Autodesk Inventor part; units mm, degrees
ref_plane "YZ Plane" through (0, 0, 0) normal (1, 0, 0) x (0, 1, 0)
ref_plane "XZ Plane" through (0, 0, 0) normal (0, 1, 0) x (-1, 0, 0)
ref_plane "XY Plane" through (0, 0, 0) normal (0, 0, 1) x (1, 0, 0)
sketch "スケッチ1" plane through (0, 0, 0) normal (1, 0, 0) x (0, 1, 0)
  circle A0 centre (0, 0) radius 14
  circle A1 centre (0, 0) radius 4
  dimension "d0" = 8
  dimension "d1" = 28
extrude "押し出し1" add sketch "スケッチ1" along normal blind 1.5
sketch "スケッチ2" plane through (1.5, 0, 0) normal (1, 0, 0) x (0, 0, -1)
  circle A0 centre (0, 0) radius 4
  circle A1 centre (0, 0) radius 7.5
  dimension "d9" = 15
extrude "押し出し2" add sketch "スケッチ2" along normal blind 2.5
sketch "スケッチ3" plane through (4, 0, 0) normal (1, 0, 0) x (0, 0, -1)
  circle A0 centre (0, 0) radius 6 construction
  line L0 (0, 0) -> (6, 0) construction
  point P0 (0, 6)
  point P1 (-6, 0)
  point P2 (0, -6)
  dimension "d12" = 12
  dimension "d15" = 360
hole "穴1" at (4, 0, -6) at (4, 6, 0) at (4, 0, 6) at (4, -6, 0) direction (-1, 0, 0) diameter 1.5 end through all both
sketch "スケッチ4" plane through (4, 0, 0) normal (1, 0, 0) x (0, 0, -1)
  line L0 (0, 0) -> (4.2426, 4.2426) construction
  circle A0 centre (0, 0) radius 6 construction
  line L1 (0, 0) -> (12.9289, 0) construction
  point P0 (-4.2426, 4.2426)
  point P1 (-4.2426, -4.2426)
  point P2 (4.2426, -4.2426)
  dimension "d25" = 12
  dimension "d24" = 45
  dimension "d28" = 360
hole "穴2" at (4, 4.2426, -4.2426) at (4, 4.2426, 4.2426) at (4, -4.2426, 4.2426) at (4, -4.2426, -4.2426) direction (-1, 0, 0) diameter 1.567 end through all
sketch "スケッチ7" plane through (1.5, 0, 0) normal (1, 0, 0) x (0, 0, -1)
  circle A0 centre (0, 0) radius 8.4
  circle A1 centre (0, 0) radius 10.2
  dimension "d37" = 16.8
  dimension "d48" = 20.4
extrude "押し出し3" cut sketch "スケッチ7" against normal blind 0.2
sketch "スケッチ8" plane through (1.5, 0, 0) normal (1, 0, 0) x (0, 0, -1)
  circle A0 centre (0, 0) radius 12 construction
  circle A1 centre (0, 0) radius 12.55
  circle A2 centre (0, 0) radius 11.45
  dimension "d40" = 24
  dimension "d41" = 0.55
  dimension "d42" = 0.55
extrude "押し出し4" cut sketch "スケッチ8" against normal blind 0.5
chamfer "面取り1" distance 0.25 angle 45 1 edges at (1.5, -14, 0)
properties part number "COXA_PITCH_BEARING_BASE"
Could you check a few things on this model? Use its own coordinates, in mm. A direction names the side the tool comes from. Coordinates: 2 decimals unless noted, no trailing zeros. Put each result on its own line as item: value. Start each with the question number.
(1) I need wall thicknesses on line 1 (Y direction, x = 2.7, z = 0); line 2 (Z direction, x = 1.3, y = 10.5); line 3 (Z direction, x = 0.9, y = -0.5). Which ranges of each line are inside material? Lowest first, please. Write a range as from..to.
(2) Suppose I cut it at A-A on x = 2. Count the separate pieces of the cut face and the enclosed holes in it, then the cut area to 3 significant figures.
(3) Will this pin go through, and if not, where does the flat tip stop? P1, Ø1.4, axis at y = 4.24, z = 4.24, coming from the -X side (3 decimals).
(4) For faces 1 (the face through (1.972, 4.007, 3.495)), 2 (the face through (1, -6, -10)), which set-ups out of +Z, -Z, +X, -X, +Y, -Y let a thin tool reach every point of the face, with its end or its side?
(5) Thinking about a two-plate mould opening in Z: for faces 3 (the face through (0.616, 12.932, 5.362)), 4 (the face through (1.97, -0.03, 6.75)), 5 (the face through (0, 3, -3)), which applies, pulls with the +Z half, pulls with the -Z half, needs draft (parallel to the pull), parting line crosses it, or undercut?
Solutions:
1. line 1: y = -7.5..-6.75, -5.25..-4, 4..5.25, 6.75..7.5
1. line 2: z = -9.18..-6.87, -4.57..4.57, 6.87..9.18
1. line 3: z = -13.99..-6.56, -5.44..-3.97, 3.97..5.44, 6.56..13.99
2. separate pieces: 1
2. enclosed holes: 9
2. area: 112 mm2
3. P1: passes through
4. face 1: +X, -X
4. face 2: +X
5. face 3: parting line crosses it
5. face 4: undercut
5. face 5: needs draft
